from build123d import *

# Parameters (mm, degrees)
SKETCH1_W                    = 88.9
SKETCH1_H                    = 38.1
BOSS_EXTRUDE1_DEPTH          = 1016
SHELL1_T                     = -6.35
F_5_16_1_66_DIAMETER_HOLE1_D = 42.164


with BuildPart() as part:
    # Sketch1 → Boss-Extrude1 (new body)
    with BuildSketch(Plane(origin=(0, 0, 0), x_dir=(0, 1, 0), z_dir=(0, 0, 1))):
        Rectangle(SKETCH1_W, SKETCH1_H)
    extrude(amount=BOSS_EXTRUDE1_DEPTH)

    # Shell1
    shell1_openings = [part.faces().sort_by_distance(p)[0] for p in [
        (0, 0, 0),
    ]]
    offset(amount=SHELL1_T, openings=shell1_openings, kind=Kind.INTERSECTION)

    # 5/16 (1.66) Diameter Hole1 (through all)
    with Locations(Plane.YZ.offset(19.05)):
        with Locations((0, 685.8)):
            Hole(F_5_16_1_66_DIAMETER_HOLE1_D / 2)


solid = part.part
Part model, mm, in its own coordinate system. A direction names the side the tool comes from. Round coordinates to 2 decimals unless told otherwise and drop trailing zeros. Write each loop counter-clockwise with the first axis right and the second up, starting at its lowest first coordinate (ties: lowest second). Pieces come first, ordered by that corner, then holes. Notation, with made-up numbers: M 80,38.25 L 108,38.25 A20 cw 108,61.25 Z; hole C 53,-2.75 d10. An arc over 180 degrees is marked long. Return JSON: item names as keys, results as strings. Group by question number.
(1) Pin check, flat tips, straight feed: pin 1 Ø8 at (x, y) = (1.5, -6) entering from -Z; pin 2 Ø20.5 at (x, y) = (-2.5, 19) entering from -Z. Stop position of each tip, or through.
(2) Which spindle directions (+Z, -Z, +X, -X, +Y, -Y) get a long thin tool onto all of the face, cutting with end or side? Do faces 5 (the face through (12.7, -1, 498)), 6 (the face through (0, 44.45, 501)). Say none if no direction does.
(3) Drill centre lines: probe 1 along X at (y, z) = (25, 166.5); probe 2 along Z at (x, y) = (-14.5, 0); probe 3 along Y at (x, z) = (4, 608.5). Where is each one in solid material? Low to high.
(4) Saw through at B-B on z = 685.8. Write the cut outline in (x, y), then the cut area to 3 significant figures.
(5) Saw through at D-D on x = 3. Write the cut outline in (y, z), then the cut area to 3 significant figures.
(6) Two-plate mould, pull along X, no slides. Class faces 1 (the face through (-19.05, -1, 501)), 2 (the face through (0, -38.1, 498)), 3 (the face through (-13, -1, 0)), 4 (the face through (0, -1, 1009.65)): +X half, -X half, draft (parallel to the pull), parting line (faces both ways), or undercut.
(7) Saw through at C-C on z = 331.5. Write the cut outline in (x, y), then the cut area to 3 significant figures.
(8) Saw through at A-A on y = 0. Write the cut outline in (x, z), then the cut area to 3 significant figures.
Returned:
{
 "1": {"pin 1": "z = 1009.65", "pin 2": "z = 0"},
 "2": {"face 5": "-Z", "face 6": "+Z, -Z, +X, -X, +Y"},
 "3": {"probe 1": "-19.05 to -12.7, 12.7 to 19.05", "probe 2": "0 to 664.72, 706.88 to 1016", "probe 3": "-44.45 to -38.1, 38.1 to 44.45"},
 "4": {"outline": "M -19.05,-44.45 L 19.05,-44.45 L 19.05,-21.08 L 12.7,-21.08 L 12.7,-38.1 L -12.7,-38.1 L -12.7,-21.08 L -19.05,-21.08 Z; M -19.05,21.08 L -12.7,21.08 L -12.7,38.1 L 12.7,38.1 L 12.7,21.08 L 19.05,21.08 L 19.05,44.45 L -19.05,44.45 Z", "area": "916 mm²"},
 "5": {"outline": "M -44.45,0 L -38.1,0 L -38.1,1009.65 L 38.1,1009.65 L 38.1,0 L 44.45,0 L 44.45,1016 L -44.45,1016 Z", "area": "13,400 mm²"},
 "6": {"face 1": "-X half", "face 2": "undercut", "face 3": "draft", "face 4": "undercut"},
 "7": {"outline": "M -19.05,-44.45 L 19.05,-44.45 L 19.05,44.45 L -19.05,44.45 Z; hole M -12.7,-38.1 L 12.7,-38.1 L 12.7,38.1 L -12.7,38.1 Z", "area": "1,450 mm²"},
 "8": {"outline": "M -19.05,0 L -12.7,0 L -12.7,664.72 L -19.05,664.72 Z; M -19.05,706.88 L -12.7,706.88 L -12.7,1009.65 L 12.7,1009.65 L 12.7,706.88 L 19.05,706.88 L 19.05,1016 L -19.05,1016 Z; M 12.7,0 L 19.05,0 L 19.05,664.72 L 12.7,664.72 Z", "area": "12,500 mm²"}
}
